Read the model definition and answer for the solid it produces. Units are mm, in the model's axes. Give positions to 0.01 mm unless a question says otherwise; leave off trailing zeros. Order: outer loops, then holes, each group sorted by start corner. A loop starts at its lowest first (then second) coordinate and runs counter-clockwise, first axis right, second up.
Item 1: A cutting plane is placed at C-C (y = 1.65). State how many separate pieces and enclosed holes the cut face has, plus the area to 3 significant figures.
Item 2: A cutting plane is placed at A-A (x = 128). Write down the section's boundary in (y, z), plus the area to 3 significant figures.
Item 3: Find the intervals of material crossed by line 1 along X through (y, z) = (2.95, -31); line 2 along Z through (x, y) = (180.88, 1.7); line 3 along Z through (x, y) = (194, 4.1), in increasing order.
Item 4: A cutting plane is placed at B-B (z = -40). Write down the section's boundary in (x, y), plus the area to 3 significant figures.
from build123d import *

# Parameters (mm, degrees)
SKETCH1_R           = 1.5
SKETCH1_W           = 30
SKETCH1_H           = 5
SKETCH1_W_2         = 5
SKETCH1_H_2         = 50
SKETCH1_W_3         = 60
SKETCH1_H_3         = 100
BOSS_EXTRUDE1_DEPTH = 5


with BuildPart() as part:
    # Sketch1 → Boss-Extrude1 (new body)
    # profile 1 of 2: a face of its own
    with BuildSketch(Plane(origin=(0, 0, 0), x_dir=(1, 0, 0), z_dir=(0, 1, 0))):
        with BuildLine():
            ThreePointArc((0, 10), (2.928932188, 2.928932188), (10, 0))
            Line((10, 0), (240, 0))
            ThreePointArc((240, 0), (247.071067812, 2.928932188), (250, 10))
            Line((250, 10), (250, 340))
            ThreePointArc((250, 340), (247.071067812, 347.071067812), (240, 350))
            Line((240, 350), (10, 350))
            ThreePointArc((10, 350), (2.928932188, 347.071067812), (0, 340))
            Line((0, 340), (0, 10))
        make_face()
        with Locations(Location((17, 17, 0), (0, 0, 270))):
            Circle(SKETCH1_R, mode=Mode.SUBTRACT)
        with Locations((42, 9.5)):
            Rectangle(SKETCH1_W, SKETCH1_H, mode=Mode.SUBTRACT)
        with Locations((9.5, 52)):
            Rectangle(SKETCH1_W_2, SKETCH1_H_2, mode=Mode.SUBTRACT)
        with Locations(Location((45.15, 110, 0), (0, 0, 270))):
            Circle(SKETCH1_R, mode=Mode.SUBTRACT)
        with Locations(Location((115, 110, 0), (0, 0, 270))):
            Circle(SKETCH1_R, mode=Mode.SUBTRACT)
        with Locations((125, 9.5)):
            Rectangle(SKETCH1_W_3, SKETCH1_H, mode=Mode.SUBTRACT)
        with Locations((208, 9.5)):
            Rectangle(SKETCH1_W, SKETCH1_H, mode=Mode.SUBTRACT)
        with Locations(Location((233, 17, 0), (0, 0, 270))):
            Circle(SKETCH1_R, mode=Mode.SUBTRACT)
        with Locations((240.5, 52)):
            Rectangle(SKETCH1_W_2, SKETCH1_H_2, mode=Mode.SUBTRACT)
        with Locations(Location((135, 110, 0), (0, 0, 270))):
            Circle(SKETCH1_R, mode=Mode.SUBTRACT)
        with Locations(Location((204.85, 110, 0), (0, 0, 270))):
            Circle(SKETCH1_R, mode=Mode.SUBTRACT)
        Polygon((7, 175), (7, 225), (12, 225), (12, 125), (7, 125), align=None, mode=Mode.SUBTRACT)
        with Locations(Location((17, 206, 0), (0, 0, 270))):
            Circle(SKETCH1_R, mode=Mode.SUBTRACT)
        with Locations(Location((45.15, 179.98, 0), (0, 0, 270))):
            Circle(SKETCH1_R, mode=Mode.SUBTRACT)
        with Locations(Location((69.12, 213.48, 0), (0, 0, 270))):
            Circle(SKETCH1_R, mode=Mode.SUBTRACT)
        with Locations(Location((115, 179.98, 0), (0, 0, 270))):
            Circle(SKETCH1_R, mode=Mode.SUBTRACT)
        with Locations((9.5, 298)):
            Rectangle(SKETCH1_W_2, SKETCH1_H_2, mode=Mode.SUBTRACT)
        with Locations(Location((17, 333, 0), (0, 0, 270))):
            Circle(SKETCH1_R, mode=Mode.SUBTRACT)
        with Locations((42, 340.5)):
            Rectangle(SKETCH1_W, SKETCH1_H, mode=Mode.SUBTRACT)
        with Locations(Location((69.12, 310, 0), (0, 0, 270))):
            Circle(SKETCH1_R, mode=Mode.SUBTRACT)
        with Locations(Location((135, 179.98, 0), (0, 0, 270))):
            Circle(SKETCH1_R, mode=Mode.SUBTRACT)
        with Locations(Location((180.88, 213.48, 0), (0, 0, 270))):
            Circle(SKETCH1_R, mode=Mode.SUBTRACT)
        with Locations(Location((204.85, 179.98, 0), (0, 0, 270))):
            Circle(SKETCH1_R, mode=Mode.SUBTRACT)
        with Locations((240.5, 175)):
            Rectangle(SKETCH1_W_2, SKETCH1_H_3, mode=Mode.SUBTRACT)
        with Locations(Location((233, 206, 0), (0, 0, 270))):
            Circle(SKETCH1_R, mode=Mode.SUBTRACT)
        Polygon((95, 343), (125, 343), (155, 343), (155, 338), (95, 338), align=None, mode=Mode.SUBTRACT)
        with Locations(Location((180.88, 310, 0), (0, 0, 270))):
            Circle(SKETCH1_R, mode=Mode.SUBTRACT)
        with Locations((240.5, 298)):
            Rectangle(SKETCH1_W_2, SKETCH1_H_2, mode=Mode.SUBTRACT)
        with Locations((208, 340.5)):
            Rectangle(SKETCH1_W, SKETCH1_H, mode=Mode.SUBTRACT)
        with Locations(Location((233, 333, 0), (0, 0, 270))):
            Circle(SKETCH1_R, mode=Mode.SUBTRACT)
    # profile 2 of 2: a face of its own
    with BuildSketch(Plane(origin=(0, 0, 0), x_dir=(1, 0, 0), z_dir=(0, 1, 0))):
        with BuildLine():
            ThreePointArc((0, 10), (2.928932188, 2.928932188), (10, 0))
            Line((10, 0), (240, 0))
            ThreePointArc((240, 0), (247.071067812, 2.928932188), (250, 10))
            Line((250, 10), (250, 340))
            ThreePointArc((250, 340), (247.071067812, 347.071067812), (240, 350))
            Line((240, 350), (10, 350))
            ThreePointArc((10, 350), (2.928932188, 347.071067812), (0, 340))
            Line((0, 340), (0, 10))
        make_face()
        with Locations(Location((17, 17, 0), (0, 0, 270))):
            Circle(SKETCH1_R, mode=Mode.SUBTRACT)
        with Locations((42, 9.5)):
            Rectangle(SKETCH1_W, SKETCH1_H, mode=Mode.SUBTRACT)
        with Locations((9.5, 52)):
            Rectangle(SKETCH1_W_2, SKETCH1_H_2, mode=Mode.SUBTRACT)
        with Locations(Location((45.15, 110, 0), (0, 0, 270))):
            Circle(SKETCH1_R, mode=Mode.SUBTRACT)
        with Locations(Location((115, 110, 0), (0, 0, 270))):
            Circle(SKETCH1_R, mode=Mode.SUBTRACT)
        with Locations((125, 9.5)):
            Rectangle(SKETCH1_W_3, SKETCH1_H, mode=Mode.SUBTRACT)
        with Locations((208, 9.5)):
            Rectangle(SKETCH1_W, SKETCH1_H, mode=Mode.SUBTRACT)
        with Locations(Location((233, 17, 0), (0, 0, 270))):
            Circle(SKETCH1_R, mode=Mode.SUBTRACT)
        with Locations((240.5, 52)):
            Rectangle(SKETCH1_W_2, SKETCH1_H_2, mode=Mode.SUBTRACT)
        with Locations(Location((135, 110, 0), (0, 0, 270))):
            Circle(SKETCH1_R, mode=Mode.SUBTRACT)
        with Locations(Location((204.85, 110, 0), (0, 0, 270))):
            Circle(SKETCH1_R, mode=Mode.SUBTRACT)
        Polygon((7, 175), (7, 225), (12, 225), (12, 125), (7, 125), align=None, mode=Mode.SUBTRACT)
        with Locations(Location((17, 206, 0), (0, 0, 270))):
            Circle(SKETCH1_R, mode=Mode.SUBTRACT)
        with Locations(Location((45.15, 179.98, 0), (0, 0, 270))):
            Circle(SKETCH1_R, mode=Mode.SUBTRACT)
        with Locations(Location((69.12, 213.48, 0), (0, 0, 270))):
            Circle(SKETCH1_R, mode=Mode.SUBTRACT)
        with Locations(Location((115, 179.98, 0), (0, 0, 270))):
            Circle(SKETCH1_R, mode=Mode.SUBTRACT)
        with Locations((9.5, 298)):
            Rectangle(SKETCH1_W_2, SKETCH1_H_2, mode=Mode.SUBTRACT)
        with Locations(Location((17, 333, 0), (0, 0, 270))):
            Circle(SKETCH1_R, mode=Mode.SUBTRACT)
        with Locations((42, 340.5)):
            Rectangle(SKETCH1_W, SKETCH1_H, mode=Mode.SUBTRACT)
        with Locations(Location((69.12, 310, 0), (0, 0, 270))):
            Circle(SKETCH1_R, mode=Mode.SUBTRACT)
        with Locations(Location((135, 179.98, 0), (0, 0, 270))):
            Circle(SKETCH1_R, mode=Mode.SUBTRACT)
        with Locations(Location((180.88, 213.48, 0), (0, 0, 270))):
            Circle(SKETCH1_R, mode=Mode.SUBTRACT)
        with Locations(Location((204.85, 179.98, 0), (0, 0, 270))):
            Circle(SKETCH1_R, mode=Mode.SUBTRACT)
        with Locations((240.5, 175)):
            Rectangle(SKETCH1_W_2, SKETCH1_H_3, mode=Mode.SUBTRACT)
        with Locations(Location((233, 206, 0), (0, 0, 270))):
            Circle(SKETCH1_R, mode=Mode.SUBTRACT)
        Polygon((95, 343), (125, 343), (155, 343), (155, 338), (95, 338), align=None, mode=Mode.SUBTRACT)
        with Locations(Location((180.88, 310, 0), (0, 0, 270))):
            Circle(SKETCH1_R, mode=Mode.SUBTRACT)
        with Locations((240.5, 298)):
            Rectangle(SKETCH1_W_2, SKETCH1_H_2, mode=Mode.SUBTRACT)
        with Locations((208, 340.5)):
            Rectangle(SKETCH1_W, SKETCH1_H, mode=Mode.SUBTRACT)
        with Locations(Location((233, 333, 0), (0, 0, 270))):
            Circle(SKETCH1_R, mode=Mode.SUBTRACT)
    extrude(amount=BOSS_EXTRUDE1_DEPTH)


solid = part.part
Response values:
1. separate pieces: 1
1. enclosed holes: 30
1. area: 84,100 mm2
2. outline: (0, -350) - (5, -350) - (5, -343) - (0, -343) - close; (0, -338) - (5, -338) - (5, -12) - (0, -12) - close; (0, -7) - (5, -7) - (5, 0) - (0, 0) - close
2. area: 1,700 mm2
3. line 1: x = 0 to 7, 12 to 238, 243 to 250
3. line 2: z = -350 to -311.5, -308.5 to -214.98, -211.98 to 0
3. line 3: z = -350 to -343, -338 to -12, -7 to 0
4. outline: (0, 0) - (7, 0) - (7, 5) - (0, 5) - close; (12, 0) - (238, 0) - (238, 5) - (12, 5) - close; (243, 0) - (250, 0) - (250, 5) - (243, 5) - close
4. area: 1,200 mm2
